Build history of the part. All positions in model axes, mm. A direction names the side the tool comes from. Round coordinates to 2 decimals unless told otherwise and drop trailing zeros. Write each loop counter-clockwise with the first axis right and the second up, starting at its lowest first coordinate (ties: lowest second). Pieces come first, ordered by that corner, then holes. Notation, with made-up numbers: M 69,75.25 L 111,75.25 A16 cw 111,79.25 Z; hole C 15,76 d11. An arc over 180 degrees is marked long. Write item = value, one per line.
from build123d import *

# Parameters (mm, degrees)
SKETCH2_W                    = 47.5
SKETCH2_H                    = 15
CUT_EXTRUDE1_DEPTH           = 79.846369606
F_7_0_7_DIAMETER_HOLE1_D     = 7
F_7_0_7_DIAMETER_HOLE1_DEPTH = 10
M6X1_0_TAPPED_HOLE1_REACH    = 100.969
M6X1_0_TAPPED_HOLE1_BORE_R   = 2.5
CIRPATTERN1_COUNT            = 2
CIRPATTERN1_ANGLE            = 120


with BuildPart() as part:
    # Sketch1 → Revolve1 (revolve)
    with BuildSketch(Plane(origin=(0, 0, 0), x_dir=(0, 0, -1), z_dir=(1, 0, 0)), mode=Mode.PRIVATE) as revolve1_sk:
        Polygon((-47.5, 34.5), (-46.5, 34.5), (-46.5, 40.055), (-47.5, 44.5), (-45.5, 44.5), (-44.5, 40.055), (-3, 40.055), (-2, 44.5), (0, 44.5), (-1, 40.055), (-1, 34.5), (0, 34.5), (0, 0), (-47.5, 0), align=None)
    revolve(revolve1_sk.sketch.rotate(Axis((0, 0, 52.856940479), (0, 0, -1)), 90), axis=Axis((0, 0, 52.856940479), (0, 0, -1)))

    # Sketch2 → Cut-Revolve1 (revolve, cut)
    with BuildSketch(Plane(origin=(0, 0, 0), x_dir=(0, 0, -1), z_dir=(1, 0, 0)), mode=Mode.PRIVATE) as cut_revolve1_sk:
        with Locations((-23.75, 7.5)):
            Rectangle(SKETCH2_W, SKETCH2_H)
    revolve(cut_revolve1_sk.sketch.rotate(Axis((0, 0, -27.972108766), (0, 0, 1)), 90), axis=Axis((0, 0, -27.972108766), (0, 0, 1)), mode=Mode.SUBTRACT)

    # Sketch3 → Cut-Extrude1 (cut, through all)
    with BuildSketch(Plane.XY.offset(47.5)):
        with BuildLine():
            Line((-4, 18.3), (4, 18.3))
            Line((4, 18.3), (4, 14.456832295))
            ThreePointArc((4, 14.456832295), (0, 15), (-4, 14.456832295))
            Line((-4, 14.456832295), (-4, 18.3))
        make_face()
    extrude(amount=-CUT_EXTRUDE1_DEPTH, mode=Mode.SUBTRACT)

    # Ø7.0 (7) Diameter Hole1
    with Locations(Plane(origin=(0, 40.055, 0), x_dir=(-1, 0, 0), z_dir=(0, 1, 0))):
        with Locations((0, 23.75)):
            f_7_0_7_diameter_hole1 = Hole(F_7_0_7_DIAMETER_HOLE1_D / 2, depth=F_7_0_7_DIAMETER_HOLE1_DEPTH)

    # M6x1.0 Tapped Hole1 bore → M6x1.0 Tapped Hole1 (cut, up to next)
    with BuildSketch(Plane(origin=(0, 30.055, 0), x_dir=(-1, 0, 0), z_dir=(0, 1, 0)), mode=Mode.PRIVATE) as m6x1_0_tapped_hole1_sk1:
        with Locations((0, 23.75)):
            Circle(M6X1_0_TAPPED_HOLE1_BORE_R)
    m6x1_0_tapped_hole1_tool1 = extrude(m6x1_0_tapped_hole1_sk1.sketch, amount=-M6X1_0_TAPPED_HOLE1_REACH, mode=Mode.PRIVATE) & part.part
    m6x1_0_tapped_hole1 = m6x1_0_tapped_hole1_tool1.solids().sort_by_distance((0, 30.055, 23.75))[0]
    add(m6x1_0_tapped_hole1, mode=Mode.SUBTRACT)

    # CirPattern1: Ø7.0 (7) Diameter Hole1, M6x1.0 Tapped Hole1; each copy of M6x1.0 Tapped Hole1 runs up to whatever stops it at its own place
    cirpattern1_before = part.part  # the part as the pattern finds it: every copy runs up to it
    add(f_7_0_7_diameter_hole1.rotate(Axis((0, 0, -27.972108766), (0, 0, 1)), 1 * CIRPATTERN1_ANGLE / (CIRPATTERN1_COUNT - 1)), mode=Mode.SUBTRACT)
    cirpattern1_m6x1_0_tapped_hole1_long = extrude(m6x1_0_tapped_hole1_sk1.sketch, amount=-M6X1_0_TAPPED_HOLE1_REACH, mode=Mode.PRIVATE)
    cirpattern1_m6x1_0_tapped_hole1_tool1 = cirpattern1_m6x1_0_tapped_hole1_long.rotate(Axis((0, 0, -27.972108766), (0, 0, 1)), 1 * CIRPATTERN1_ANGLE / (CIRPATTERN1_COUNT - 1)) & cirpattern1_before
    add(cirpattern1_m6x1_0_tapped_hole1_tool1.solids().sort_by_distance((-26.028394, -15.0275, 23.75))[0], mode=Mode.SUBTRACT)


solid = part.part
1. Mould opens along X. For faces 1 (the face through (-32.798, -30.075, 0.986)), 2 (the face through (7, 15, 0)), 3 (the face through (-34.467, -1.517, 46.993)) say: pulls with the +X half, pulls with the -X half, needs draft (parallel to the pull), parting line crosses it, or undercut.
Responses:
face_1 = parting line crosses it
face_2 = needs draft
face_3 = undercut
2. Band-saw the part on C-C (x = 0). Count the separate pieces of the cut face and the enclosed holes in it, plus the area to 3 significant figures.
Responses:
separate_pieces = 3
enclosed_holes = 0
area = 2,110 mm²
3. Tool access for faces 4 (the face through (-4, 16, 24)), 5 (the face through (18, -30, 1)), 6 (the face through (18.61, 35.78, 2.94)), 7 (the face through (-18, -30, 46.5)): list every direction of +Z, -Z, +X, -X, +Y, -Y with a clear straight run to the whole face (end or side of a thin tool).
Responses:
face_4 = +Z, -Z
face_5 = -Z
face_6 = none
face_7 = +Z
4. Flat gauge pins, fed straight in: pin 1 (8 mm diameter, centred on x = 0, z = 23.75, fed in from +Y) (3 decimals); pin 2 (6 mm diameter, centred on y = 3, z = 31.5, fed in from -X) (3 decimals); pin 3 (1 mm diameter, centred on x = -30.5, z = 36, fed in from -Y). Where does each tip first touch, or does it go through?
Responses:
pin_1 = 40.055
pin_2 = -40.055
pin_3 = -26.54
5. Probe probe 1 along Y at (x, z) = (0.5, 27) (3 decimals); probe 2 along Z at (x, y) = (14, 36.5); probe 3 along Z at (x, y) = (36.5, -19). List the from-to ranges inside material, lowest first.
Responses:
probe_1 = -40.052 to -14.992, 18.3 to 30.055
probe_2 = 1 to 46.5
probe_3 = 0.75 to 2.75, 44.75 to 46.75
6. Band-saw the part on B-B (z = 23.75). List the corners of the cut face in (x, y) (3 decimals).
Responses:
outline = M -36.306,-16.92 L -27.778,-11.996 L -27.278,-12.862 L -14.059,-5.23 A15 cw -4,14.457 L -4,18.3 L -2.5,18.3 L -2.5,30.055 L -3.5,30.055 L -3.5,39.902 A40.055 ccw Z; M -32.806,-22.982 A40.055 ccw long 3.5,39.902 L 3.5,30.055 L 2.5,30.055 L 2.5,18.3 L 4,18.3 L 4,14.457 A15 cw long -11.559,-9.56 L -24.778,-17.193 L -24.278,-18.059 Z
7. Band-saw the part on A-A (y = 0). List the corners of the cut face in (x, z) (3 decimals).
Responses:
outline = M -44.5,0 L -40.055,1 L -34.5,1 L -34.5,0 L -15,0 L -15,47.5 L -34.5,47.5 L -34.5,46.5 L -40.055,46.5 L -44.5,47.5 L -44.5,45.5 L -40.055,44.5 L -40.055,3 L -44.5,2 Z; M 15,0 L 34.5,0 L 34.5,1 L 40.055,1 L 44.5,0 L 44.5,2 L 40.055,3 L 40.055,44.5 L 44.5,45.5 L 44.5,47.5 L 40.055,46.5 L 34.5,46.5 L 34.5,47.5 L 15,47.5 Z
8. Band-saw the part on D-D (z = 34.5). List the corners of the cut face in (x, y) (3 decimals), plus the area to 3 significant figures.
Responses:
outline = C 0,0 d80.11; hole M -4,14.457 A15 ccw long 4,14.457 L 4,18.3 L -4,18.3 Z
area = 4,310 mm²
